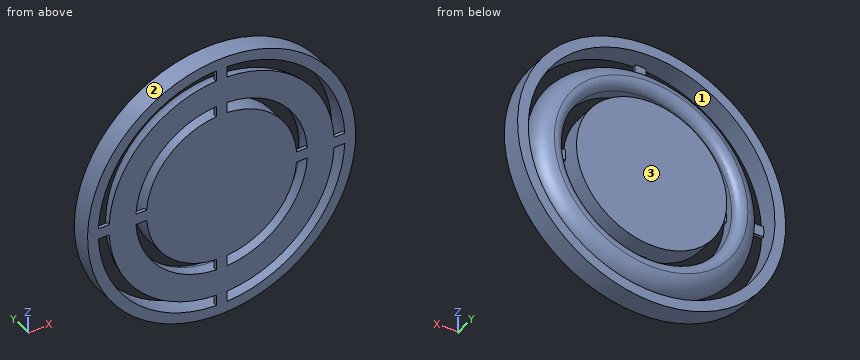
from build123d import *

# Parameters (mm, degrees)
SKETCH1_R           = 105
SKETCH1_R_2         = 80
BOSS_EXTRUDE1_DEPTH = 19.05
FILLET4_R           = 8
SKETCH6_W           = 10
SKETCH6_H           = 114.826624275
BOSS_EXTRUDE2_DEPTH = 3
CIRPATTERN2_COUNT   = 4
SKETCH5_R           = 124.826624275
SKETCH5_R_2         = 114.826624275
SKETCH5_R_3         = 70
BOSS_EXTRUDE3_DEPTH = 19.05


with BuildPart() as part:
    # Sketch1 → Boss-Extrude1 (new body)
    with BuildSketch(Plane(origin=(0, 0, 0), x_dir=(1, 0, 0), z_dir=(0, 1, 0))):
        with Locations(Location((0, 0, 0), (0, 0, 90))):
            Circle(SKETCH1_R)
        with Locations(Location((0, 0, 0), (0, 0, 90))):
            Circle(SKETCH1_R_2, mode=Mode.SUBTRACT)
    extrude(amount=BOSS_EXTRUDE1_DEPTH)

    # Sketch3 → Cut-Revolve1 (revolve, cut)
    with BuildSketch(Plane.XY, mode=Mode.PRIVATE) as cut_revolve1_sk:
        with BuildLine():
            Line((-84.849199516, 19.05), (-84.849199516, 24.05))
            Line((-84.849199516, 24.05), (-110, 24.05))
            Line((-110, 24.05), (-110, 0))
            Line((-110, 0), (-104.826624275, 0))
            ThreePointArc((-104.826624275, 0), (-98.651373258, 13.524114826), (-84.849199516, 19.05))
        make_face()
    revolve(cut_revolve1_sk.sketch.rotate(Axis((0, 0, 0), (0, 1, 0)), 270), axis=Axis((0, 0, 0), (0, 1, 0)), mode=Mode.SUBTRACT)

    # Fillet4
    fillet4_edges = [part.edges().sort_by_distance(p)[0] for p in [
        (0, 19.05, 80),
    ]]
    fillet(fillet4_edges, radius=FILLET4_R)

    # Sketch6 → Boss-Extrude2 (add)
    with BuildSketch(Plane(origin=(0, 0, 0), x_dir=(1, 0, 0), z_dir=(0, 1, 0))):
        with Locations((0, 57.413312138)):
            Rectangle(SKETCH6_W, SKETCH6_H)
    boss_extrude2 = extrude(amount=BOSS_EXTRUDE2_DEPTH)

    # CirPattern2: Boss-Extrude2 ×4 about axis
    cirpattern2_axis = Axis((0, 0, 0), (0, 1, 0))
    for i in range(1, CIRPATTERN2_COUNT):
        add(boss_extrude2.rotate(cirpattern2_axis, i * 360 / CIRPATTERN2_COUNT))

    # Sketch5 → Boss-Extrude3 (add)
    # profile 1 of 2: a face of its own
    with BuildSketch(Plane(origin=(0, 0, 0), x_dir=(1, 0, 0), z_dir=(0, 1, 0))):
        with Locations(Location((0, 0, 0), (0, 0, 90))):
            Circle(SKETCH5_R)
        with Locations(Location((0, 0, 0), (0, 0, 87.504328744))):
            Circle(SKETCH5_R_2, mode=Mode.SUBTRACT)
    # profile 2 of 2: a face of its own
    with BuildSketch(Plane(origin=(0, 0, 0), x_dir=(1, 0, 0), z_dir=(0, 1, 0))):
        with Locations(Location((0, 0, 0), (0, 0, 85.903956242))):
            Circle(SKETCH5_R_3)
    extrude(amount=BOSS_EXTRUDE3_DEPTH)


solid = part.part
Check sheet for the modelled part. Datum: model origin and axes. Units: mm. Face numbers are marked on the shaded views. Round coordinates to 2 decimals unless told otherwise and drop trailing zeros. Loops run counter-clockwise (first coordinate to the right, second up) from the corner with the lowest first, then second, coordinate; pieces in that order, holes last. Notation, with made-up numbers: (-29.5, -25.75) -> (10.5, -25.75) arc R25 ccw to (10.5, -9.75) -> close; hole circle Ø1 at (9.5, 39.5). An arc over 180 degrees is marked (long way). Put each result on its own line as item: value. Start each with the question number.
1. Gauge pin test, flat ends, axial feed: pin 1 (3 mm diameter, centred on x = -75.5, z = -2, fed in from +Y); pin 2 (2.5 mm diameter, centred on x = -76, y = 1, fed in from -Z); pin 3 (8 mm diameter, centred on y = 14.5, z = -52.5, fed in from -X). Record the tip position at first contact, or that the pin passes through.
2. Section check B-B (z = -31). Give the number of separate pieces and of enclosed holes in the cut face, plus the area to 3 significant figures.
3. Section check A-A (x = 108.5). Enter the section's corners in (y, z), plus the area to 3 significant figures.
4. Draft check along Z on the marked faces 1, 2 and 3. Enter one of: +Z half, -Z half, draft (parallel to the pull), parting line (faces both ways), or undercut.
5. Scan lines: probe 1 along X at (y, z) = (3.5, 36.5); probe 2 along Z at (x, y) = (-6.5, 13.5); probe 3 along X at (y, z) = (10, -22). Record each from-to range of solid material in increasing order.
Findings:
1. pin 1: stops at y = 3
1. pin 2: stops at z = -99.97
1. pin 3: stops at x = -115.02
2. separate pieces: 5
2. enclosed holes: 0
2. area: 3,570 mm^2
3. outline: (0, -61.72) -> (19.05, -61.72) -> (19.05, -37.59) -> (0, -37.59) -> close; (0, -5) -> (3, -5) -> (3, 5) -> (0, 5) -> close; (0, 37.59) -> (19.05, 37.59) -> (19.05, 61.72) -> (0, 61.72) -> close
3. area: 949 mm^2
4. face 1: undercut
4. face 2: parting line
4. face 3: draft
5. probe 1: x = -119.37 to -108.87, -97.76 to -71.19, -59.73 to 59.73, 71.19 to 97.76, 108.87 to 119.37
5. probe 2: z = -124.66 to -114.64, -98.46 to -80.27, -69.7 to 69.7, 80.27 to 98.46, 114.64 to 124.66
5. probe 3: x = -122.87 to -112.7, -99.17 to -76.92, -66.45 to 66.45, 76.92 to 99.17, 112.7 to 122.87
